The listing builds one solid part. Answer for the finished solid, in the listing's coordinates (mm). Face numbers are marked on the shaded views. A direction names the side the tool comes from. Coordinates: 2 decimals unless noted, no trailing zeros. Order: outer loops, then holes, each group sorted by start corner. A loop starts at its lowest first (then second) coordinate and runs counter-clockwise, first axis right, second up. Notation, with made-up numbers: (33, 9.5) -> (81, 9.5) arc R21 cw to (81, 31.5) -> close; hole circle Ø5 at (43, -1). An arc over 180 degrees is marked (long way). Return JSON: item names as keys, results as strings.
from build123d import *

# Parameters (mm, degrees)
F0_W     = 443.345444
F0_H     = 76.2
F1_DEPTH = 76.2
F2_T     = -5.08


with BuildPart() as f1:
    # F0 (on Top) → F1 (new body)
    with BuildSketch(Plane.XY):
        Rectangle(F0_W, F0_H)
    extrude(amount=F1_DEPTH)

    # F2
    f2_openings = [f1.faces().sort_by_distance(p)[0] for p in [
        (0, 0, 76.2),
        (-221.672722, 0, 38.1),
        (221.672722, 0, 38.1),
    ]]
    offset(amount=F2_T, openings=f2_openings)


solid = f1.part
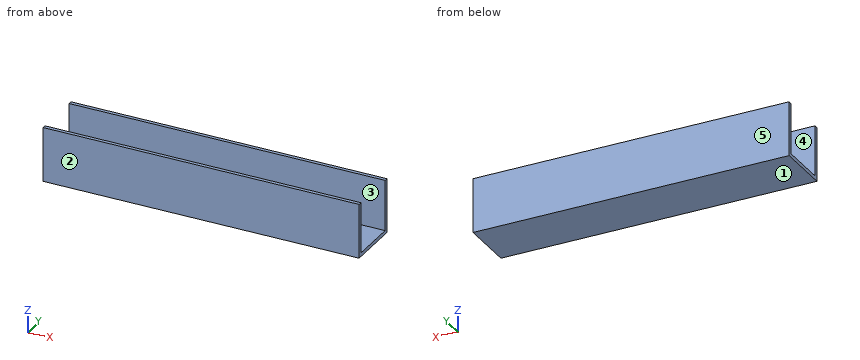
1. The part is cut by section B-B on x = 94.5. Give the vertices of the cut face in (y, z), and give its area (3 significant figures).
Answer block:
{"outline": "(-38.1, 0) -> (38.1, 0) -> (38.1, 76.2) -> (33.02, 76.2) -> (33.02, 5.08) -> (-33.02, 5.08) -> (-33.02, 76.2) -> (-38.1, 76.2) -> close", "area": "1,110 mm2"}
2. For the marked faces 4 and 5, determine the directions among +Z, -Z, +X, -X, +Y, -Y from which every point of the face is accessible in a straight line to the end or side of a thin tool.
Answer block:
{"face 4": "+Z, +X, -X", "face 5": "+Z, -Z, +X, -X, +Y"}
3. Each of these flat-tipped pins is pushed along its axis until it touches: pin 1 Ø10 at (y, z) = (23.5, 28) entering from +X; pin 2 Ø1 at (x, y) = (-10, 6) entering from +Z. Where does it stop, or does it pass through?
Answer block:
{"pin 1": "passes through", "pin 2": "stops at z = 5.08"}
4. The part is cut by section C-C on y = 21.5. Give the vertices of the cut face in (x, z), and give its area (3 significant figures).
Answer block:
{"outline": "(-221.67, 0) -> (221.67, 0) -> (221.67, 5.08) -> (-221.67, 5.08) -> close", "area": "2,250 mm2"}
5. Consider line 1 (Y direction, x = -183, z = 54.5); line 2 (Z direction, x = 123.5, y = 7). Determine where each line is inside the solid, lowest interval first. Write a range as from..to.
Answer block:
{"line 1": "y = -38.1..-33.02, 33.02..38.1", "line 2": "z = 0..5.08"}
6. Determine the mould class of the marked faces 1, 2 and 3 for opening direction Y: pulls with the +Y half, pulls with the -Y half, needs draft (parallel to the pull), parting line crosses it, or undercut.
Answer block:
{"face 1": "needs draft", "face 2": "pulls with the -Y half", "face 3": "undercut"}
7. The part is cut by section A-A on z = 68. Give the vertices of the cut face in (x, y).
Answer block:
{"outline": "(-221.67, -38.1) -> (221.67, -38.1) -> (221.67, -33.02) -> (-221.67, -33.02) -> close; (-221.67, 33.02) -> (221.67, 33.02) -> (221.67, 38.1) -> (-221.67, 38.1) -> close"}
